from build123d import *

# Parameters (mm, degrees)
SKETCH1_W           = 21
SKETCH1_H           = 21
BOSS_EXTRUDE1_DEPTH = 30
SKETCH2_R           = 4
CUT_EXTRUDE1_DEPTH  = 39.095275298
SKETCH3_R           = 4
CUT_EXTRUDE2_DEPTH  = 39.095275298


with BuildPart() as part:
    # Sketch1 → Boss-Extrude1 (new body)
    with BuildSketch(Plane(origin=(0, 0, 0), x_dir=(1, 0, 0), z_dir=(0, 1, 0))):
        Rectangle(SKETCH1_W, SKETCH1_H)
    extrude(amount=BOSS_EXTRUDE1_DEPTH)

    # Sketch2 → Cut-Extrude1 (cut, through all)
    with BuildSketch(Plane.XY.offset(10.5)):
        with Locations((0, 20)):
            Circle(SKETCH2_R)
    extrude(amount=-CUT_EXTRUDE1_DEPTH, mode=Mode.SUBTRACT)

    # Sketch3 → Cut-Extrude2 (cut, through all)
    with BuildSketch(Plane(origin=(10.5, 0, 0), x_dir=(0, 0, -1), z_dir=(1, 0, 0))):
        with Locations((0, 10)):
            Circle(SKETCH3_R)
    extrude(amount=-CUT_EXTRUDE2_DEPTH, mode=Mode.SUBTRACT)


solid = part.part
CAD build for the part. Positions are in the model's coordinates, mm. Give positions to 0.01 mm unless a question says otherwise; leave off trailing zeros. Order: outer loops, then holes, each group sorted by start corner. A loop starts at its lowest first (then second) coordinate and runs counter-clockwise, first axis right, second up. Notation, with made-up numbers: (44, 0.5) -> (62, 0.5) arc R30 cw to (62, 25.5) -> close; hole circle Ø5 at (43, 37). An arc over 180 degrees is marked (long way). Return JSON: item names as keys, results as strings.
Q1. Saw through at B-B (z = 0). Write the cut outline in (x, y).
Working result:
{"outline": "(-10.5, 0) -> (10.5, 0) -> (10.5, 6) -> (-10.5, 6) -> close; (-10.5, 14) -> (10.5, 14) -> (10.5, 30) -> (-10.5, 30) -> close; hole circle Ø8 at (0, 20)"}
Q2. Drill centre lines: line 1 (Y direction, x = 0, z = 1); line 2 (Y direction, x = -8, z = -0.25); line 3 (X direction, y = 19.75, z = 6.75). Where is each one in solid material? Low to high.
Working result:
{"line 1": "0 to 6.13, 13.87 to 16, 24 to 30", "line 2": "0 to 6.01, 13.99 to 30", "line 3": "-10.5 to -3.99, 3.99 to 10.5"}
Q3. Saw through at D-D (x = -5.75). Write the cut outline in (y, z), then the cut area to 3 significant figures.
Working result:
{"outline": "(0, -10.5) -> (30, -10.5) -> (30, 10.5) -> (0, 10.5) -> close; hole circle Ø8 at (10, 0)", "area": "580 mm²"}
Q4. Saw through at A-A (x = 0). Write the cut outline in (y, z).
Working result:
{"outline": "(0, -10.5) -> (16, -10.5) -> (16, 10.5) -> (0, 10.5) -> close; (24, -10.5) -> (30, -10.5) -> (30, 10.5) -> (24, 10.5) -> close; hole circle Ø8 at (10, 0)"}
Q5. Mould opens along Y. For faces 1 (the face through (0, 15, 10.5)), 2 (the face through (0, 0, 0)), 3 (the face through (0.147, 13.966, 0.521)) say: pulls with the +Y half, pulls with the -Y half, needs draft (parallel to the pull), parting line crosses it, or undercut.
Working result:
{"face 1": "needs draft", "face 2": "pulls with the -Y half", "face 3": "undercut"}
Q6. Flat gauge pin, fed straight in: pin 1 (1 mm diameter, centred on x = 2.5, z = 6, fed in from -Y). Where does the tip first touch, or does it go through?
Working result:
{"pin 1": "y = 0"}
Q7. Saw through at C-C (y = 10). Write the cut outline in (x, z), then the cut area to 3 significant figures.
Working result:
{"outline": "(-10.5, -10.5) -> (10.5, -10.5) -> (10.5, -4) -> (-10.5, -4) -> close; (-10.5, 4) -> (10.5, 4) -> (10.5, 10.5) -> (-10.5, 10.5) -> close", "area": "273 mm²"}
